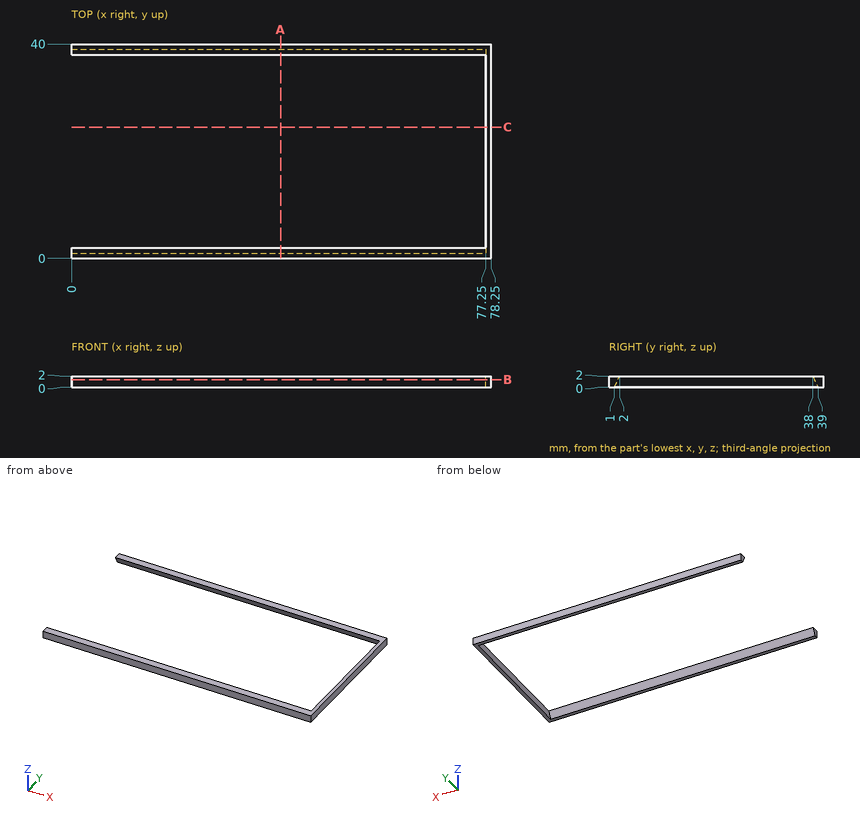
Verification items for this drawing (mm, ordinates from the low corner). Coordinates: 2 decimals unless noted, no trailing zeros. Order: outer loops, then holes, each group sorted by start corner. A loop starts at its lowest first (then second) coordinate and runs counter-clockwise, first axis right, second up. Notation, with made-up numbers: (78.5, 37.25) -> (124.5, 37.25) arc R16 ccw to (124.5, 52.25) -> close; hole circle Ø10 at (78, -8). An arc over 180 degrees is marked (long way). Put each result on its own line as item: value. Start each with the question number.
1. Cross-section at B-B, the plane z = 1.4. Record the boundary of the cut face in (x, y), then the cut area to 3 significant figures.
2. Cross-section at C-C, the plane y = 24.5. Record the boundary of the cut face in (x, z).
3. Material ranges on L1, parallel to X at y = 8, z = 0.3; L2, parallel to Y at x = 35, z = 1.5; L3, parallel to Y at x = 5, z = 0.6, recorded low to high. Write a range as [from, to].
4. Cross-section at A-A, the plane x = 39. Record the boundary of the cut face in (y, z), then the cut area to 3 significant figures.
5. Go/stop test with a flat-tipped pin: pin 1 Ø12 at (x, y) = (32, 10) entering from -Z. Record where the tip stops, or that it passes through.
Computed:
1. outline: (0, 0) -> (78.25, 0) -> (78.25, 40) -> (0, 40) -> (0, 38.3) -> (77.25, 38.3) -> (77.25, 1.7) -> (0, 1.7) -> close
1. area: 303 mm2
2. outline: (77.25, 0) -> (78.25, 0) -> (78.25, 2) -> (77.25, 2) -> close
3. L1: [77.25, 78.25]
3. L2: [0, 1.75], [38.25, 40]
3. L3: [0, 1.3], [38.7, 40]
4. outline: (0, 0) -> (1, 0) -> (2, 2) -> (0, 2) -> close; (38, 2) -> (39, 0) -> (40, 0) -> (40, 2) -> close
4. area: 6.00 mm2
5. pin 1: through
